Check sheet for the modelled part. Datum: model origin and axes. Units: mm. A direction names the side the tool comes from. Round coordinates to 2 decimals unless told otherwise and drop trailing zeros. Loops run counter-clockwise (first coordinate to the right, second up) from the corner with the lowest first, then second, coordinate; pieces in that order, holes last. Notation, with made-up numbers: (-37, 73) -> (19, 73) arc R23 cw to (19, 103) -> close; hole circle Ø6 at (25, 17.25). An arc over 180 degrees is marked (long way). One line per item, written item: value. Start each with the question number.
1. Go/stop test with flat-tipped pins: pin 1 (10 mm diameter, centred on x = 26, z = -27, fed in from -Y); pin 2 (2.5 mm diameter, centred on y = 12, z = -13.5, fed in from +X); pin 3 (7.5 mm diameter, centred on x = 199, z = -17, fed in from +Y); pin 4 (1 mm diameter, centred on y = 13, z = -13, fed in from -X). Record where each tip stops, or that it passes through.
2. Release check for a two-part mould opening along Z. For faces 1 (the face through (108, 13, -5)), 2 (the face through (113.4, 15, -25.2)), 3 (the face through (101, 7, -30)) record: +Z half, -Z half, draft (parallel to the pull), parting line (faces both ways), or undercut.
3. Material ranges on L1, parallel to Y at x = 115, z = -11; L2, parallel to Z at x = 143.5, y = 12; L3, parallel to Y at x = 215, z = -10, recorded low to high.
4. Set-up check for faces 4 (the face through (33.93, 12.54, -23.5)), 5 (the face through (187.5, 2.46, -15.16)), 6 (the face through (27.5, 12.54, -15.16)), 7 (the face through (201, 10, -15)): record each of +Z, -Z, +X, -X, +Y, -Y from which the full face is reachable in a straight line by a thin tool's end or side.
5. Cross-section at A-A on x = 160. Record the cut outline in (y, z).
from build123d import *

# Parameters (mm, degrees)
BOSS_EXTRUDE1_DEPTH = 15
CUT_EXTRUDE1_DEPTH  = 5
CUT_EXTRUDE2_DEPTH  = 5
SKETCH4_R           = 0.75
CUT_EXTRUDE3_DEPTH  = 30
CUT_EXTRUDE4_DEPTH  = 5


with BuildPart() as part:
    # Sketch1 → Boss-Extrude1 (new body)
    with BuildSketch(Plane(origin=(0, 0, 0), x_dir=(1, 0, 0), z_dir=(0, 1, 0))):
        Polygon((0, 0), (230, 0), (200, 30), (0, 30), align=None)
    extrude(amount=BOSS_EXTRUDE1_DEPTH)

    # Sketch2 → Cut-Extrude1 (cut)
    with BuildSketch(Plane(origin=(0, 15, 0), x_dir=(1, 0, 0), z_dir=(0, 1, 0))):
        with BuildLine():
            Line((-20, 22.5), (20, 22.5))
            ThreePointArc((20, 22.5), (27.5, 15), (20, 7.5))
            Line((20, 7.5), (-20, 7.5))
            ThreePointArc((-20, 7.5), (-27.5, 15), (-20, 22.5))
        make_face()
        with BuildLine():
            Line((235, 22.5), (195, 22.5))
            ThreePointArc((195, 22.5), (187.5, 15), (195, 7.5))
            Line((195, 7.5), (235, 7.5))
            ThreePointArc((235, 7.5), (242.5, 15), (235, 22.5))
        make_face()
    extrude(amount=-CUT_EXTRUDE1_DEPTH, mode=Mode.SUBTRACT)

    # Sketch3 → Cut-Extrude2 (cut)
    with BuildSketch(Plane.XZ):
        with BuildLine():
            Line((195, -7.5), (222.5, -7.5))
            Line((222.5, -7.5), (207.5, -22.5))
            Line((207.5, -22.5), (195, -22.5))
            ThreePointArc((195, -22.5), (187.5, -15), (195, -7.5))
        make_face()
        with BuildLine():
            Line((0, -22.5), (0, -7.5))
            Line((0, -7.5), (20, -7.5))
            ThreePointArc((20, -7.5), (27.5, -15), (20, -22.5))
            Line((20, -22.5), (0, -22.5))
        make_face()
    extrude(amount=-CUT_EXTRUDE2_DEPTH, mode=Mode.SUBTRACT)

    # Sketch4 → Cut-Extrude3 (cut)
    with BuildSketch(Plane.XY):
        with Locations((115, 7.5)):
            Circle(SKETCH4_R)
        with Locations((165, 7.5)):
            Circle(SKETCH4_R)
        with Locations((215, 7.5)):
            Circle(SKETCH4_R)
        with Locations((65, 7.5)):
            Circle(SKETCH4_R)
        with Locations((15, 7.5)):
            Circle(SKETCH4_R)
    extrude(amount=-CUT_EXTRUDE3_DEPTH, mode=Mode.SUBTRACT)

    # Sketch5 → Cut-Extrude4 (cut)
    with BuildSketch(Plane(origin=(0, 15, 0), x_dir=(1, 0, 0), z_dir=(0, 1, 0))):
        with BuildLine():
            Line((37.5, 25), (177.5, 25))
            ThreePointArc((177.5, 25), (181.035533906, 23.535533906), (182.5, 20))
            Line((182.5, 20), (182.5, 10))
            ThreePointArc((182.5, 10), (181.035533906, 6.464466094), (177.5, 5))
            Line((177.5, 5), (37.5, 5))
            ThreePointArc((37.5, 5), (33.964466094, 6.464466094), (32.5, 10))
            Line((32.5, 10), (32.5, 20))
            ThreePointArc((32.5, 20), (33.964466094, 23.535533906), (37.5, 25))
        make_face()
    extrude(amount=-CUT_EXTRUDE4_DEPTH, mode=Mode.SUBTRACT)


solid = part.part
Taken from the geometry:
1. pin 1: stops at y = 0
1. pin 2: stops at x = 188.02
1. pin 3: stops at y = 10
1. pin 4: stops at x = 27.07
2. face 1: undercut
2. face 2: draft
2. face 3: -Z half
3. L1: y = 0 to 6.75, 8.25 to 10
3. L2: z = -30 to -25, -5 to 0
3. L3: y = 5 to 6.75, 8.25 to 10
4. face 4: +Y
4. face 5: +X, -Y
4. face 6: -X, +Y
4. face 7: +X, +Y
5. outline: (0, -30) -> (15, -30) -> (15, -25) -> (10, -25) -> (10, -5) -> (15, -5) -> (15, 0) -> (0, 0) -> close
